```python
from build123d import *

# Parameters (mm, degrees)
F1_DEPTH = 10
F3_DEPTH = 25
F4_W     = 439.603239
F4_H     = 26.46663
F4_H_2   = 44.717323
F4_H_3   = 46.259694
F4_H_4   = 33.076853
F5_DEPTH = 5


with BuildPart() as f1:
    # F0 (on Front) → F1 (new body)
    with BuildSketch(Plane.XZ):
        with BuildLine():
            Line((494.592618, 316.358934), (-465.407382, 316.358934))
            ThreePointArc((-465.407382, 316.358934), (-479.549518, 310.501069), (-485.407382, 296.358934))
            Line((-485.407382, 296.358934), (-485.407382, -163.641066))
            ThreePointArc((-485.407382, -163.641066), (-479.549518, -177.783202), (-465.407382, -183.641066))
            Line((-465.407382, -183.641066), (494.592618, -183.641066))
            ThreePointArc((494.592618, -183.641066), (508.734753, -177.783202), (514.592618, -163.641066))
            Line((514.592618, -163.641066), (514.592618, 296.358934))
            ThreePointArc((514.592618, 296.358934), (508.734753, 310.501069), (494.592618, 316.358934))
        make_face()
    extrude(amount=F1_DEPTH)

    # F2 (on face) → F3 (cut)
    with BuildSketch(Plane.XZ.offset(10)):
        with BuildLine():
            Line((453.451734, 267.632127), (50.635236, 267.632127))
            ThreePointArc((50.635236, 267.632127), (36.4931, 261.774262), (30.635236, 247.632127))
            Line((30.635236, 247.632127), (30.635236, -121.80623))
            ThreePointArc((30.635236, -121.80623), (36.4931, -135.948366), (50.635236, -141.80623))
            Line((50.635236, -141.80623), (453.451734, -141.80623))
            ThreePointArc((453.451734, -141.80623), (467.593869, -135.948366), (473.451734, -121.80623))
            Line((473.451734, -121.80623), (473.451734, 247.632127))
            ThreePointArc((473.451734, 247.632127), (467.593869, 261.774262), (453.451734, 267.632127))
        make_face()
    extrude(amount=-F3_DEPTH, mode=Mode.SUBTRACT)

    # F4 (on face) → F5 (cut)
    with BuildSketch(Plane(origin=(0, 0, 0), x_dir=(-1, 0, 0), z_dir=(0, 1, 0))):
        with Locations((219.801619, -128.572915)):
            Rectangle(F4_W, F4_H)
        with Locations((219.801619, -22.358662)):
            Rectangle(F4_W, F4_H_2)
        with Locations((219.801619, 109.305013)):
            Rectangle(F4_W, F4_H_3)
        with Locations((219.801619, 251.0937)):
            Rectangle(F4_W, F4_H_4)
    extrude(amount=-F5_DEPTH, mode=Mode.SUBTRACT)


solid = f1.part
```
Read the model definition and answer for the solid it produces. Units are mm, in the model's axes. A direction names the side the tool comes from. Coordinates: 2 decimals unless noted, no trailing zeros. Loops run counter-clockwise (first coordinate to the right, second up) from the corner with the lowest first, then second, coordinate; pieces in that order, holes last.
(1) A flat-ended cylindrical pin translates along its axis: pin 1 Ø10 at (x, z) = (-291, 259) entering from +Y. Find the tip coordinate at first contact, or state that the pin passes through.
Solution:
pin 1: stops at y = -5
(2) The part is cut by section A-A (x = 98.5). Determine the outline of the cut face in (y, z).
Solution:
outline: (-10, -183.64) - (0, -183.64) - (0, -141.81) - (-10, -141.81) - close; (-10, 267.63) - (0, 267.63) - (0, 316.36) - (-10, 316.36) - close
(3) The part is cut by section B-B (z = -27). Determine the outline of the cut face in (x, y), and give its area (3 significant figures).
Solution:
outline: (-485.41, -10) - (30.64, -10) - (30.64, 0) - (0, 0) - (0, -5) - (-439.6, -5) - (-439.6, 0) - (-485.41, 0) - close; (473.45, -10) - (514.59, -10) - (514.59, 0) - (473.45, 0) - close
area: 3,370 mm2
(4) The part is cut by section C-C (y = -2). Count the separate pieces of the cut face and the enclosed holes in it, and give its area (3 significant figures).
Solution:
separate pieces: 1
enclosed holes: 5
area: 253,000 mm2
(5) Consider line 1 along Z through (x, y) = (-22, -1.5); line 2 along X through (y, z) = (-7, 154.5); line 3 along Z through (x, y) = (244, -1). Determine where each line is inside the solid, lowest interval first.
Solution:
line 1: z = -183.64 to -141.81, -115.34 to -44.72, 0 to 86.18, 132.43 to 234.56, 267.63 to 316.36
line 2: x = -485.41 to 30.64, 473.45 to 514.59
line 3: z = -183.64 to -141.81, 267.63 to 316.36
(6) The mould has two halves that part along X. Classify faces 1 (the face through (467.749, -5.07, 261.618)), 2 (the face through (508.578, -4.93, -177.938)), 3 (the face through (-104, -10, 70)): released by +X, released by -X, zero draft, split by the parting line, or undercut.
Solution:
face 1: undercut
face 2: released by +X
face 3: zero draft
(7) The part is cut by section D-D (x = -247). Determine the outline of the cut face in (y, z), and give its area (3 significant figures).
Solution:
outline: (-10, -183.64) - (0, -183.64) - (0, -141.81) - (-5, -141.81) - (-5, -115.34) - (0, -115.34) - (0, -44.72) - (-5, -44.72) - (-5, 0) - (0, 0) - (0, 86.18) - (-5, 86.18) - (-5, 132.43) - (0, 132.43) - (0, 234.56) - (-5, 234.56) - (-5, 267.63) - (0, 267.63) - (0, 316.36) - (-10, 316.36) - close
area: 4,250 mm2
(8) A tool of negligible diameter and unlimited length cuts with its end or side. For faces 4 (the face through (36.338, -5.07, -135.792)), 5 (the face through (-217, -5, 110)), 6 (the face through (-479.39, -4.93, 310.66)), from which of +Z, -Z, +X, -X, +Y, -Y can it reach the whole face along a straight path? Write none if from no direction.
Solution:
face 4: +Y, -Y
face 5: +Y
face 6: +Z, -X, +Y, -Y
